Verification items for the finished model (mm, model axes). A direction names the side the tool comes from. Coordinates: 2 decimals unless noted, no trailing zeros. Order: outer loops, then holes, each group sorted by start corner. A loop starts at its lowest first (then second) coordinate and runs counter-clockwise, first axis right, second up. Notation, with made-up numbers: (-32, 10.25) - (23, 10.25) arc R23 cw to (23, 38.25) - close; hole circle Ø2 at (52, 72.5). An arc over 180 degrees is marked (long way). Answer as CSV lines item,"result". Start each with the question number.
1. Material ranges on L1, parallel to Y at x = 40, z = 37; L2, parallel to Y at x = 25, z = 45; L3, parallel to Z at x = 28.5, y = 14, recorded low to high. Write a range as [from, to].
2. Section check B-B (z = 44.5). Record the cut outline in (x, y).
3. Set-up check for faces 5 (the flat face through (31.788, 15.492, 55.394)), 6 (the flat face through (31.79, -19.66, 51.65)): record each of +Z, -Z, +X, -X, +Y, -Y from which the full face is reachable in a straight line by a thin tool's end or side.
4. Section check C-C (y = 11). Record the cut outline in (x, z).
5. Mould release check, pull along Y, two halves, no side actions. Record for faces 1 (the flat face through (31.788, 9.489, 10.888)), 2 (the flat face through (0, 5, 37)), 3 (the flat face through (31.79, -9.49, 57.24)), 4 (the flat face through (31.8, -12.9, 25.2)): pulls with the +Y half, pulls with the -Y half, needs draft (parallel to the pull), parting line crosses it, or undercut.
6. Go/stop test with flat-tipped pins: pin 1 (1.5 mm diameter, centred on x = 9.5, z = 46.5, fed in from -Y); pin 2 (12 mm diameter, centred on x = 18.5, z = 21.5, fed in from +Y); pin 3 (5 mm diameter, centred on x = 40.5, y = 19, fed in from -Z); pin 4 (8 mm diameter, centred on y = 9, z = 34, fed in from -X). Record where each tip stops, or that it passes through.
7. Section check A-A (x = 45). Record the cut outline in (y, z).
from build123d import *

# Parameters (mm, degrees)
F2_DEPTH = 64.478658


with BuildPart() as f2:
    # F1 (on face) → F2 (new body)
    with BuildSketch(Plane.YZ):
        Polygon((30.557144, 59.066296), (0, 51.617414), (-19.239661, 63.016182), (-20.095591, 39.965741), (-5.539023, 10.089733), (24.94307, 11.708565), align=None)
    extrude(amount=F2_DEPTH)


solid = f2.part
Evaluation:
1,L1,"y = [-18.65, 27.94]"
1,L2,"y = [-19.91, 28.89]"
1,L3,"z = [11.13, 55.03]"
2,outline,"(0, -19.93) - (64.48, -19.93) - (64.48, 28.83) - (0, 28.83) - close"
3,face 5,"+Z, +X, -X"
3,face 6,"+Z, +X, -X, -Y"
4,outline,"(0, 10.97) - (64.48, 10.97) - (64.48, 54.3) - (0, 54.3) - close"
5,face 1,"pulls with the +Y half"
5,face 2,"needs draft"
5,face 3,"undercut"
5,face 4,"pulls with the -Y half"
6,pin 1,"stops at y = -19.88"
6,pin 2,"stops at y = 26.82"
6,pin 3,"stops at z = 11.26"
6,pin 4,"stops at x = 0"
7,outline,"(-20.1, 39.97) - (-5.54, 10.09) - (24.94, 11.71) - (30.56, 59.07) - (0, 51.62) - (-19.24, 63.02) - close"
